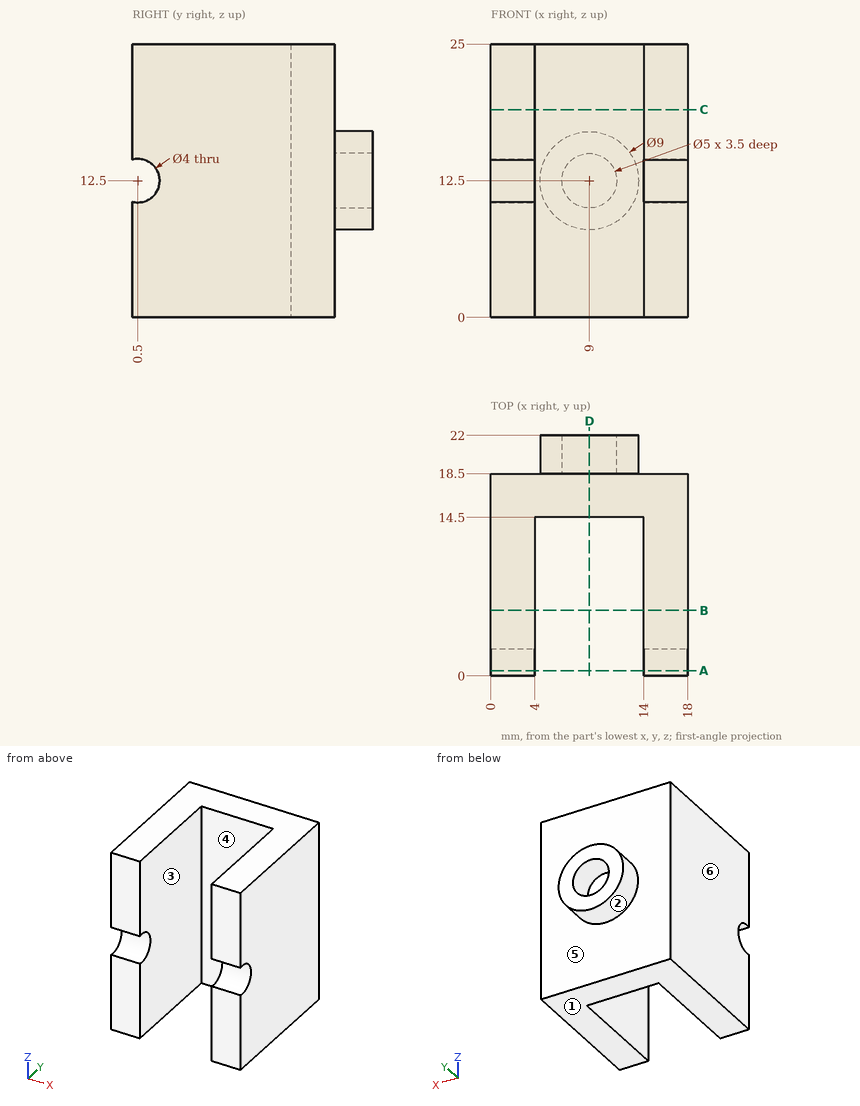
Answer from the drawing. Dimensions are ordinates in mm from the lowest x, y and z of the part. A direction names the side the tool comes from. Coordinates: 2 decimals unless noted, no trailing zeros. Order: outer loops, then holes, each group sorted by start corner. A loop starts at its lowest first (then second) coordinate and runs counter-clockwise, first axis right, second up. Notation, with made-up numbers: (28.25, 48.5) - (72.25, 48.5) arc R17 ccw to (72.25, 79.5) - close; hole circle Ø7 at (10.25, 22.25). An arc over 180 degrees is marked (long way). Use one line per item in the form item = value.
(1) Section B-B, the plane y = 6 is taken. Give the vertices of the cut face in (x, z), then the cut area to 3 significant figures.
Computed values:
outline = (0, 0) - (4, 0) - (4, 25) - (0, 25) - close; (14, 0) - (18, 0) - (18, 25) - (14, 25) - close
area = 200 mm²
(2) Section C-C, the plane z = 19 is taken. Give the vertices of the cut face in (x, y), then the cut area to 3 significant figures.
Computed values:
outline = (0, 0) - (4, 0) - (4, 14.5) - (14, 14.5) - (14, 0) - (18, 0) - (18, 18.5) - (0, 18.5) - close
area = 188 mm²
(3) Straight lines are drawn through the part: L1, parallel to X at y = 20.25, z = 12.5; L2, parallel to X at y = 11, z = 12.25; L3, parallel to Z at x = 16.15, y = 0.5. For each, find the intervals that lie inside material, in ascending order.
Computed values:
L1 = 4.5 to 6.5, 11.5 to 13.5
L2 = 0 to 4, 14 to 18
L3 = 0 to 10.5, 14.5 to 25
(4) Section D-D, the plane x = 9 is taken. Give the vertices of the cut face in (y, z).
Computed values:
outline = (14.5, 0) - (18.5, 0) - (18.5, 8) - (22, 8) - (22, 10) - (18.5, 10) - (18.5, 15) - (22, 15) - (22, 17) - (18.5, 17) - (18.5, 25) - (14.5, 25) - close
(5) For a pull along X with two mould halves and no side action, classify the marked faces 4, 5 and 6 as pulls with the +X half, pulls with the -X half, needs draft (parallel to the pull), parting line crosses it, or undercut.
Computed values:
face_4 = undercut
face_5 = needs draft
face_6 = pulls with the -X half
(6) Given pin 1 Ø4 at (x, z) = (9, 12.5) entering from +Y, flat-ended and moving along its own axis, determine where the tip first touches the part or whether it passes through.
Computed values:
pin_1 = 18.5
(7) Section A-A, the plane y = 0.5 is taken. Give the vertices of the cut face in (x, z).
Computed values:
outline = (0, 0) - (4, 0) - (4, 10.5) - (0, 10.5) - close; (0, 14.5) - (4, 14.5) - (4, 25) - (0, 25) - close; (14, 0) - (18, 0) - (18, 10.5) - (14, 10.5) - close; (14, 14.5) - (18, 14.5) - (18, 25) - (14, 25) - close
(8) Which of the six approach directions +Z, -Z, +X, -X, +Y, -Y give full straight-line access (tool end or side, diameter ignored) to the marked faces 1, 2 and 3?
Computed values:
face_1 = -Z, +X, -X, +Y, -Y
face_2 = +Y
face_3 = +Z, -Z, -Y
